from build123d import *

# Parameters (mm, degrees)
SWEEP1_PROFILE_R        = 16.7005
SHELL1_T                = -3.556
F_1_4_CLEARANCE_HOLE4_D = 7.14248


with BuildPart() as part:
    # Sweep1: sweep along a path in Sketch2
    with BuildLine(Plane(origin=(0, 0, 0), x_dir=(0, 0, -1), z_dir=(1, 0, 0))) as sweep1_path:
        Line((0, 0), (0, 609.6))
    # Sweep1 profile (on start of the path) → Sweep1 (sweep)
    with BuildSketch(Plane.ZX):
        Circle(SWEEP1_PROFILE_R)
    sweep(path=sweep1_path.line)

    # Shell1
    shell1_openings = [part.faces().sort_by_distance(p)[0] for p in [
        (0, 609.6, 16.7005),
        (0, 0, 16.7005),
    ]]
    offset(amount=SHELL1_T, openings=shell1_openings, kind=Kind.INTERSECTION)

    # 1/4 Clearance Hole4 (through all)
    with Locations(Plane.XY.offset(16.7005)):
        with Locations((0, 593.725)):
            Hole(F_1_4_CLEARANCE_HOLE4_D / 2)


solid = part.part
Check sheet for the modelled part. Datum: model origin and axes. Units: mm. Round coordinates to 2 decimals unless told otherwise and drop trailing zeros. Order: outer loops, then holes, each group sorted by start corner. A loop starts at its lowest first (then second) coordinate and runs counter-clockwise, first axis right, second up.
Q1. Depth check by flat-ended pin: P1, Ø12, axis at y = 454.5, z = 8, coming from the +X side; P2, Ø3, axis at y = 434.5, z = 5, coming from the +X side; P3, Ø4, axis at x = -2.5, y = 119, coming from the +Z side. Enter the tip coordinate at first touch or a pass-through.
Filled sheet:
P1: stops at x = 16.58
P2: stops at x = 16.33
P3: stops at z = 16.69
Q2. Scan lines: L1, parallel to X at y = 482, z = 1; L2, parallel to Y at x = 0, z = 15. Record each from-to range of solid material in increasing order.
Filled sheet:
L1: x = -16.67 to -13.11, 13.11 to 16.67
L2: y = 0 to 590.15, 597.3 to 609.6
Q3. Draft check along Z on faces 1 (the face through (-14, 0, 0)), 2 (the face through (3.948, 309.067, 12.538)), 3 (the face through (-16.303, 309.067, -3.62)). Enter one of: pulls with the +Z half, pulls with the -Z half, needs draft (parallel to the pull), parting line crosses it, or undercut.
Filled sheet:
face 1: needs draft
face 2: undercut
face 3: parting line crosses it
Q4. Cross-section at B-B, the plane y = 178. Enter the section's corners in (x, z).
Filled sheet:
outline: circle Ø33.4 at (0, 0); hole circle Ø26.29 at (0, 0)
Q5. Cross-section at A-A, the plane z = 0. Enter the section's corners in (x, y).
Filled sheet:
outline: (-16.7, 0) - (-13.14, 0) - (-13.14, 609.6) - (-16.7, 609.6) - close; (13.14, 0) - (16.7, 0) - (16.7, 609.6) - (13.14, 609.6) - close
